Autodesk Inventor part; units mm, degrees
ref_plane "YZ Plane" through (0, 0, 0) normal (1, 0, 0) x (0, 1, 0)
ref_plane "XZ Plane" through (0, 0, 0) normal (0, 1, 0) x (-1, 0, 0)
ref_plane "XY Plane" through (0, 0, 0) normal (0, 0, 1) x (1, 0, 0)
sketch "Sketch1" plane through (0, 0, 0) normal (0, 1, 0) x (-1, 0, 0)
  line L0 (317.5, 444.5) -> (-317.5, 444.5)
  line L1 (-317.5, 444.5) -> (-317.5, -444.5)
  line L2 (-317.5, -444.5) -> (317.5, -444.5)
  line L3 (317.5, -444.5) -> (317.5, 444.5)
  line L4 (317.5, 444.5) -> (-317.5, -444.5) construction
  line L5 (-317.5, 444.5) -> (317.5, -444.5) construction
  point P0 (0, 0)
  dimension "d0" = 635
  dimension "d1" = 889
extrude "Extrusion1" add sketch "Sketch1" against normal blind 25.4
sketch "Sketch2" plane through (0, 0, 0) normal (0, 1, 0) x (1, 0, 0)
  line L0 (-317.5, -444.5) -> (-317.5, 444.5)
  line L1 (-317.5, -241.3) -> (-266.7, -241.3)
  line L2 (-266.7, -241.3) -> (-266.7, -139.7)
  line L3 (-266.7, -139.7) -> (-317.5, -139.7)
  line L4 (-317.5, -139.7) -> (-317.5, -241.3)
  line L5 (-317.5, -444.5) -> (317.5, -444.5)
  point P0 (0, 0)
  dimension "d6" = 101.6
  dimension "d7" = 50.8
  dimension "d8" = 203.2
extrude "Extrusion2" add sketch "Sketch2" along normal blind 762
mirror "Mirror1" about plane through (0, 0, 0) normal (1, 0, 0) of "Extrusion2"
sketch "Sketch3" plane through (317.5, -25.4, 444.5) normal (1, 0, 0) x (0, 0, -1)
  line L0 (304.8, 787.4) -> (203.2, 787.4) construction
  line L1 (254, 787.4) -> (254, -228.6) construction
  circle A0 centre (254, 762) radius 12.7
  point P0 (444.5, 25.4)
  dimension "d9" = 25.4
  dimension "d10" = 25.4
extrude "Extrusion4" add sketch "Sketch3" against normal through all
equation "\"d4\" = heightOfArm"
equation "\"robotLength\" = 889"
equation "\"heightOfArm\" = 762"
properties part number "Catapult"
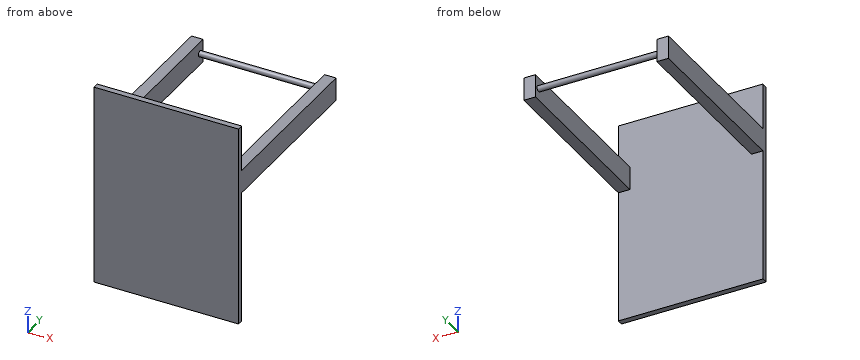
Verification items for the finished model (mm, model axes). Round coordinates to 2 decimals unless told otherwise and drop trailing zeros. Write each loop counter-clockwise with the first axis right and the second up, starting at its lowest first coordinate (ties: lowest second). Pieces come first, ordered by that corner, then holes. Notation, with made-up numbers: (46, 57) -> (99, 57) arc R14 ccw to (99, 63) -> close; hole circle Ø6 at (56.25, 78.25). An arc over 180 degrees is marked (long way). Write each question's results on one line, items separated by ' | '. Start each with the question number.
1. Cross-section at B-B (x = -72.5). Enter the section's corners in (y, z), then the cut area to 3 significant figures.
2. Depth check by flat-ended pin: P1, Ø15, axis at x = -286.5, y = 469, coming from the -Z side; P2, Ø15, axis at x = 286.5, y = 545.5, coming from the +Z side. Enter the tip coordinate at first touch or a pass-through.
3. Cross-section at C-C (z = 190.5). Enter the section's corners in (x, y).
4. Material ranges on probe 1 along Y at (x, z) = (13, -337.5); probe 2 along Z at (x, y) = (-270.5, 85.5), recorded low to high. Write a range as from..to.
5. Cross-section at A-A (y = 668). Enter the section's corners in (x, z).
Solutions:
1) outline: (-25.4, -444.5) -> (0, -444.5) -> (0, 444.5) -> (-25.4, 444.5) -> close; circle Ø25.4 at (736.6, 190.5) | area: 23,100 mm2
2) P1: stops at z = 139.7 | P2: stops at z = 241.3
3) outline: (-317.5, -25.4) -> (317.5, -25.4) -> (317.5, 762) -> (266.7, 762) -> (266.7, 749.3) -> (-266.7, 749.3) -> (-266.7, 762) -> (-317.5, 762) -> close; hole (-266.7, 0) -> (266.7, 0) -> (266.7, 723.9) -> (-266.7, 723.9) -> close
4) probe 1: y = -25.4..0 | probe 2: z = 139.7..241.3
5) outline: (-317.5, 139.7) -> (-266.7, 139.7) -> (-266.7, 241.3) -> (-317.5, 241.3) -> close; (266.7, 139.7) -> (317.5, 139.7) -> (317.5, 241.3) -> (266.7, 241.3) -> close
